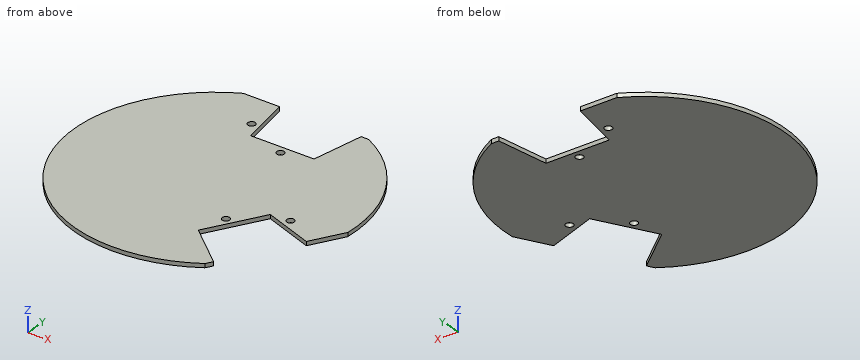
from build123d import *

# Parameters (mm, degrees)
ESQUISSE1_R             = 175
BOSS_EXTRU_1_DEPTH      = 5
ESQUISSE2_R             = 4.7
ENL_V_MAT_EXTRU_1_DEPTH = 5


with BuildPart() as part:
    # Esquisse1 → Boss.-Extru.1 (new body)
    with BuildSketch(Plane.XY):
        Circle(ESQUISSE1_R)
    extrude(amount=BOSS_EXTRU_1_DEPTH)

    # Esquisse2 → Enlèv. mat.-Extru.1 (cut)
    with BuildSketch(Plane(origin=(0, 0, 0), x_dir=(-1, 0, 0), z_dir=(0, 0, -1))):
        with Locations((-23.220426897, 80.887612711)):
            Circle(ESQUISSE2_R)
        with Locations((35.460378836, 110.887612711)):
            Circle(ESQUISSE2_R)
        with Locations((-58.440514011, -60.553285934)):
            Circle(ESQUISSE2_R)
        with Locations((-113.761678991, -24.734217455)):
            Circle(ESQUISSE2_R)
        Polygon((21.779573103, 90.887612711), (33.263317057, 156.015161015), (79.273384773, 156.015161015), (79.273384773, 185.246123659), (-115.714238566, 185.246123659), (-115.714238566, 156.015161015), (-69.70417085, 156.015161015), (-58.220426897, 90.887612711), align=None)
        Polygon((-89.600768048, -26.582142764), (-151.744751343, -49.200702922), (-174.749785201, -9.35481545), (-200.064541428, -23.970296772), (-102.570729758, -192.834532007), (-77.255973531, -178.219050686), (-100.26100739, -138.373163213), (-49.600768048, -95.864175067), align=None)
    extrude(amount=-ENL_V_MAT_EXTRU_1_DEPTH, mode=Mode.SUBTRACT)


solid = part.part
Geometry check sheet. Reference: the model listing, model coordinates, mm. Give positions to 0.01 mm unless a question says otherwise; leave off trailing zeros. Loops run counter-clockwise (first coordinate to the right, second up) from the corner with the lowest first, then second, coordinate; pieces in that order, holes last. Notation, with made-up numbers: (78.25, 59.5) -> (98.25, 59.5) arc R24 cw to (98.25, 80.5) -> close; hole circle Ø4 at (84, 0.5). An arc over 180 degrees is marked (long way). Answer in a Markdown table with one row per item. Add a question column.
1) Cross-section at D-D on x = -142.5. Record the boundary of the cut face in (y, z).
2) Cross-section at C-C on x = 0. Record the boundary of the cut face in (y, z).
3) Gauge pin test, flat ends, axial feed: P1, Ø1.5, axis at y = 87, z = 2, coming from the +X side; P2, Ø1, axis at y = 28.5, z = 4, coming from the +X side; P3, Ø11, axis at x = 113.76, y = -24.73, coming from the -Z side; P4, Ø7.5, axis at x = 58.44, y = -60.55, coming from the -Z side. Record the tip position at first contact, or that the pin passes through.
4) Material ranges on probe 1 along X at (y, z) = (-4, 1.05); probe 2 along X at (y, z) = (126.5, 2.9); probe 3 along X at (y, z) = (-2, 2.1), recorded low to high. Write a range as from..to.
5) Cross-section at B-B on y = 126. Record the boundary of the cut face in (x, z).
6) Cross-section at A-A on z = 1.05. Record the boundary of the cut face in (x, y), and give its area (3 significant figures).
Outcome:
| question | item | result |
|---|---|---|
| 1 | outline | (-101.58, 0) -> (101.58, 0) -> (101.58, 5) -> (-101.58, 5) -> close |
| 2 | outline | (-175, 0) -> (90.89, 0) -> (90.89, 5) -> (-175, 5) -> close |
| 3 | P1 | stops at x = 152.27 |
| 3 | P2 | stops at x = 172.75 |
| 3 | P3 | stops at z = 0 |
| 3 | P4 | passes through |
| 4 | probe 1 | x = -174.95..174.95 |
| 4 | probe 2 | x = -120.92..-28.06, 64.5..120.92 |
| 4 | probe 3 | x = -174.99..174.99 |
| 5 | outline | (-121.45, 0) -> (-27.97, 0) -> (-27.97, 5) -> (-121.45, 5) -> close; (64.41, 0) -> (121.45, 0) -> (121.45, 5) -> (64.41, 5) -> close |
| 6 | outline | (-79.27, 156.02) arc R175 ccw (long way) to (95.48, -146.66) -> (100.26, -138.37) -> (49.6, -95.86) -> (89.6, -26.58) -> (151.74, -49.2) -> (174.75, -9.35) arc R175 ccw to (79.27, 156.02) -> (69.7, 156.02) -> (58.22, 90.89) -> (-21.78, 90.89) -> (-33.26, 156.02) -> close; hole circle Ø9.4 at (-35.46, 110.89); hole circle Ø9.4 at (23.22, 80.89); hole circle Ø9.4 at (58.44, -60.55); hole circle Ø9.4 at (113.76, -24.73) |
| 6 | area | 80,000 mm^2 |
